from build123d import *

# Parameters (mm, degrees)
SKETCH1_R           = 2.55
BOSS_EXTRUDE1_DEPTH = 3


with BuildPart() as part:
    # Sketch1 → Boss-Extrude1 (new body)
    with BuildSketch(Plane(origin=(0, 0, 0), x_dir=(1, 0, 0), z_dir=(0, 1, 0))):
        with BuildLine():
            Line((-170, 27.5), (-170, 10.5))
            ThreePointArc((-170, 10.5), (-170.878679656, 8.378679656), (-173, 7.5))
            Line((-173, 7.5), (-290, 7.5))
            Line((-290, 7.5), (-290, -42.5))
            Line((-290, -42.5), (270, -42.5))
            Line((270, -42.5), (270, 7.5))
            Line((270, 7.5), (153, 7.5))
            ThreePointArc((153, 7.5), (150.878679656, 8.378679656), (150, 10.5))
            Line((150, 10.5), (150, 27.5))
            Line((150, 27.5), (-170, 27.5))
        make_face()
        with Locations((-250, -32.5)):
            Circle(SKETCH1_R, mode=Mode.SUBTRACT)
        with Locations((-30, -32.5)):
            Circle(SKETCH1_R, mode=Mode.SUBTRACT)
        with Locations((230, -32.5)):
            Circle(SKETCH1_R, mode=Mode.SUBTRACT)
    extrude(amount=BOSS_EXTRUDE1_DEPTH)


solid = part.part
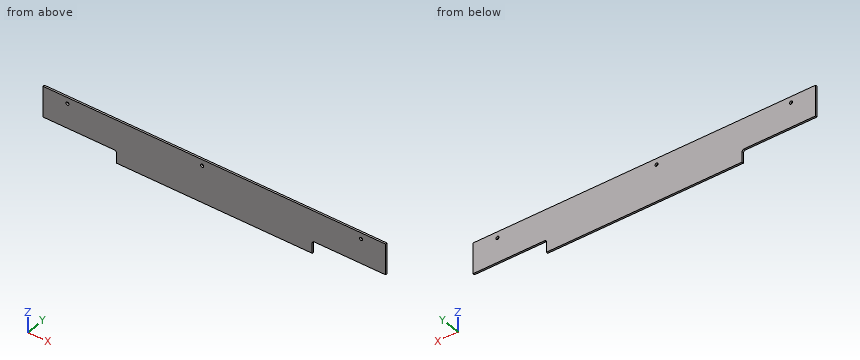
Can you work these out from the model? Positions are in its coordinate system, mm. Give positions to 0.01 mm unless a question says otherwise; leave off trailing zeros. Loops run counter-clockwise (first coordinate to the right, second up) from the corner with the lowest first, then second, coordinate; pieces in that order, holes last. Notation, with made-up numbers: (4, 66.5) - (36, 66.5) arc R24 cw to (36, 88.5) - close; hole circle Ø10 at (-26, 78.5). An arc over 180 degrees is marked (long way). Answer as a JSON object with one key per item and string values.
Q1. If I drill on L1, parallel to X at y = 1, z = 32.5; L2, parallel to Z at x = 230, y = 0.8; L3, parallel to X at y = 2.05, z = 31.5, over which ranges is the centre line in solid material (lowest first)?
Geometry says:
{"L1": "-290 to -252.55, -247.45 to -32.55, -27.45 to 227.45, 232.55 to 270", "L2": "-7.5 to 29.95, 35.05 to 42.5", "L3": "-290 to -252.35, -247.65 to -32.35, -27.65 to 227.65, 232.35 to 270"}
Q2. Imagine slicing it at A-A on y = 2.5. Write out the boundary of the cut face in (x, z).
Geometry says:
{"outline": "(-290, -7.5) - (-173, -7.5) arc R3 cw to (-170, -10.5) - (-170, -27.5) - (150, -27.5) - (150, -10.5) arc R3 cw to (153, -7.5) - (270, -7.5) - (270, 42.5) - (-290, 42.5) - close; hole circle Ø5.1 at (-250, 32.5); hole circle Ø5.1 at (-30, 32.5); hole circle Ø5.1 at (230, 32.5)"}
Q3. Will this pin go through, and if not, where does the flat tip stop? P1, Ø2, axis at x = 5.5, z = -12, coming from the -Y side.
Geometry says:
{"P1": "y = 0"}
Q4. Imagine slicing it at C-C on z = -22.5. Write out the boundary of the cut face in (x, y), plus the area to 3 significant figures.
Geometry says:
{"outline": "(-170, 0) - (150, 0) - (150, 3) - (-170, 3) - close", "area": "960 mm²"}
Q5. Imagine slicing it at B-B on x = 173.5. Write out the boundary of the cut face in (y, z), plus the area to 3 significant figures.
Geometry says:
{"outline": "(0, -7.5) - (3, -7.5) - (3, 42.5) - (0, 42.5) - close", "area": "150 mm²"}
